from build123d import *

# Parameters (mm, degrees)
CROQUIS1_W              = 32
CROQUIS1_H              = 41.37
CROQUIS1_R              = 5.3
SALIENTE_EXTRUIR1_DEPTH = 2
CROQUIS2_R              = 1.8
CORTAR_EXTRUIR1_DEPTH   = 2
MATRIZC1_COUNT          = 4
REDONDEO1_R             = 4


with BuildPart() as part:
    # Croquis1 → Saliente-Extruir1 (new body)
    with BuildSketch(Plane(origin=(0, 0, 0), x_dir=(1, 0, 0), z_dir=(0, 1, 0))):
        Rectangle(CROQUIS1_W, CROQUIS1_H)
        with Locations((-4.5, -9.565)):
            Circle(CROQUIS1_R, mode=Mode.SUBTRACT)
    extrude(amount=SALIENTE_EXTRUIR1_DEPTH)

    # Croquis2 → Cortar-Extruir1 (cut)
    with BuildSketch(Plane(origin=(0, 2, 0), x_dir=(1, 0, 0), z_dir=(0, 1, 0))):
        with Locations((2.924621202, -16.989621202)):
            Circle(CROQUIS2_R)
    cortar_extruir1 = extrude(amount=-CORTAR_EXTRUIR1_DEPTH, mode=Mode.SUBTRACT)

    # MatrizC1: Cortar-Extruir1 ×4 about axis
    matrizc1_axis = Axis((-4.5, 0, 9.565), (0, 1, 0))
    for i in range(1, MATRIZC1_COUNT):
        add(cortar_extruir1.rotate(matrizc1_axis, i * 360 / MATRIZC1_COUNT), mode=Mode.SUBTRACT)

    # Redondeo1
    redondeo1_edges = [part.edges().sort_by_distance(p)[0] for p in [
        (16, 1, 20.685),
        (-16, 1, 20.685),
        (-16, 1, -20.685),
        (16, 1, -20.685),
    ]]
    fillet(redondeo1_edges, radius=REDONDEO1_R)


solid = part.part
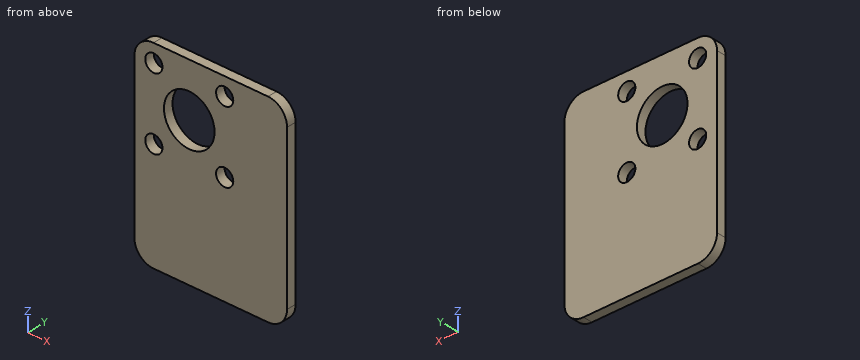
Design review of the part built by this model. Coordinates are the model's own, in mm. Round coordinates to 2 decimals unless told otherwise and drop trailing zeros. Order: outer loops, then holes, each group sorted by start corner. A loop starts at its lowest first (then second) coordinate and runs counter-clockwise, first axis right, second up. Notation, with made-up numbers: M 59,-37.5 L 75,-37.5 A29 ccw 75,1.5 Z; hole C 62.25,-19.75 d10. An arc over 180 degrees is marked long. Answer as CSV lines item,"result". Start each with the question number.
1) Add section B-B (y = 0.9). Give the boundary of the cut face in (x, z) (3 decimals), then the cut area to 3 significant figures.
2) Add section A-A (x = -5.5). Give the boundary of the cut face in (y, z) (3 decimals).
3) Wall thickness on line 1 along Z through (x, y) = (-12, 0.5) (3 decimals); line 2 along Z through (x, y) = (-4.5, 1.05) (3 decimals); line 3 along X through (y, z) = (0.7, 15.5): over which ranges is each line inside the solid? List them lowest first. Write a range as [from, to].
4) Add section C-C (x = 14). Give the boundary of the cut face in (y, z).
Resolved:
1,outline,"M -16,-16.685 A4 ccw -12,-20.685 L 12,-20.685 A4 ccw 16,-16.685 L 16,16.685 A4 ccw 12,20.685 L -12,20.685 A4 ccw -16,16.685 Z; hole C -11.925,2.14 d3.6; hole C -11.925,16.99 d3.6; hole C -4.5,9.565 d10.6; hole C 2.925,2.14 d3.6; hole C 2.925,16.99 d3.6"
1,area,"1,180 mm^2"
2,outline,"M 0,-20.685 L 2,-20.685 L 2,4.36 L 0,4.36 Z; M 0,14.77 L 2,14.77 L 2,20.685 L 0,20.685 Z"
3,line 1,"[-20.685, 0.342], [3.939, 15.191], [18.788, 20.685]"
3,line 2,"[-20.685, 4.265], [14.865, 20.685]"
3,line 3,"[-16, -12.94], [-10.91, 1.91], [3.94, 16]"
4,outline,"M 0,-20.15 L 2,-20.15 L 2,20.15 L 0,20.15 Z"
